The listing builds one solid part. Answer for the finished solid, in the listing's coordinates (mm). Face numbers are marked on the shaded views. A direction names the side the tool comes from. Round coordinates to 2 decimals unless told otherwise and drop trailing zeros. Write each loop counter-clockwise with the first axis right and the second up, starting at its lowest first coordinate (ties: lowest second). Pieces come first, ordered by that corner, then holes. Notation, with made-up numbers: (-15, 62.25) - (26, 62.25) arc R14 cw to (26, 82.25) - close; hole circle Ø5 at (43, 19.5). An arc over 180 degrees is marked (long way). Use a Markdown table: item, result. Add a question column.
1) A cutting plane is placed at D-D (y = 32.5). Give the vertices of the cut face in (x, z), then the cut area to 3 significant figures.
2) A cutting plane is placed at A-A (z = 9.75). Give the vertices of the cut face in (x, y), then the cut area to 3 significant figures.
3) Each of these flat-tipped pins is pushed along its axis until it touches: P1, Ø2.5, axis at y = 46.38, z = 14.3, coming from the -X side; P2, Ø1.8, axis at y = -14.12, z = 4.8, coming from the +X side; P3, Ø1.9, axis at y = -5.5, z = 25, coming from the -X side; P4, Ø0.8, axis at x = -25.5, z = 2, coming from the -Y side. Where does it stop, or does it pass through?
4) Determine the mould class of the marked faces 1, 2, 3 and 4 for opening direction Z: +Z half, -Z half, draft (parallel to the pull), parting line (faces both ways), or undercut.
5) A tool of negligible diameter and unlimited length cuts with its end or side. For the marked faces 5, 6, 7, 8 and 9, from which of +Z, -Z, +X, -X, +Y, -Y can it reach the whole face along a straight path? Write none if from no direction.
6) A cutting plane is placed at C-C (x = -21.5). Give the vertices of the cut face in (y, z).
7) A cutting plane is placed at B-B (x = -1). Give the vertices of the cut face in (y, z).
8) Find the intervals of material crossed by probe 1 along Y at (x, z) = (8, 24.6); probe 2 along Y at (x, z) = (-19.75, 23.8); probe 3 along X at (y, z) = (16.5, 25), in increasing order. Write a range as from..to.
```python
from build123d import *

# Parameters (mm, degrees)
EXTRUDE_1_DEPTH     = 28.6
SKETCH_1_R          = 6.5
CUT_EXTRUDE_1_DEPTH = 70.103002637
SKETCH_2_R          = 0.8
CUT_EXTRUDE_2_DEPTH = 70.103002637
CUT_EXTRUDE_4_DEPTH = 6
EXTRUDE_2_DEPTH     = 1.6
FILLET_1_R          = 1.5
FILLET_2_R          = 1.5
SKETCH_6_R          = 1.5
SKETCH_6_R_2        = 1.25
CUT_EXTRUDE_7_DEPTH = 8
CUT_EXTRUDE_8_DEPTH = 8


with BuildPart() as part:
    # Model → 凸台-拉伸1 (new body)
    with BuildSketch(Plane.XY):
        Polygon((-24.978787879, -17.92321671), (-14.678787879, -17.92321671), (-14.678787879, 24.376794113), (11.321212121, 24.376794113), (11.321212121, 51.376794114), (8.321212121, 51.376794114), (8.321212121, 28.376794114), (-23.578787879, 28.376794114), (-26.578787879, 25.376794114), (-26.578787879, 24.376794113), (-24.978787879, 24.376794113), align=None)
    extrude(amount=EXTRUDE_1_DEPTH)

    # 草图1 → 切除-拉伸1 (cut, through all)
    with BuildSketch(Plane.ZY.offset(24.978787879)):
        with Locations((14.3, -3.623205886)):
            Circle(SKETCH_1_R)
    extrude(amount=-CUT_EXTRUDE_1_DEPTH, mode=Mode.SUBTRACT)

    # 草图2 → 切除-拉伸2 (cut, through all)
    with BuildSketch(Plane.ZY.offset(24.978787879)):
        with Locations((23.8, 6.876794114)):
            Circle(SKETCH_2_R)
        with Locations((23.8, -14.123205886)):
            Circle(SKETCH_2_R)
        with Locations((4.8, -14.123205886)):
            Circle(SKETCH_2_R)
        with Locations((4.8, 6.876794114)):
            Circle(SKETCH_2_R)
    extrude(amount=-CUT_EXTRUDE_2_DEPTH, mode=Mode.SUBTRACT)

    # 草图3 → 切除-拉伸4 (cut)
    with BuildSketch(Plane.ZY.offset(24.978787879)):
        Polygon((6.3, -35.623205886), (22.3, -35.623205886), (22.3, -9.623205886), (24.3, -9.623205886), (24.3, 2.376794114), (22.3, 2.376794114), (22.3, 14.376794114), (6.3, 14.376794114), (6.3, 2.376794114), (4.3, 2.376794114), (4.3, -9.623205886), (6.3, -9.623205886), align=None)
    extrude(amount=-CUT_EXTRUDE_4_DEPTH, mode=Mode.SUBTRACT)

    # 草图5 → 凸台-拉伸2 (add, through all)
    with BuildSketch(Plane.ZY.offset(24.978787879)):
        Polygon((0, 24.376794113), (28.6, 24.376794113), (28.6, 10.676804938), (22.3, 10.676804938), (22.3, 14.376794114), (6.3, 14.376794114), (6.3, 10.676804938), (0, 10.676804938), align=None)
    extrude(amount=EXTRUDE_2_DEPTH)

    # 圆角1
    fillet_1_edges = [part.edges().sort_by_distance(p)[0] for p in [
        (-21.978787879, -9.623205886, 4.3),
        (-21.978787879, 2.376794114, 4.3),
        (-21.978787879, 2.376794114, 24.3),
        (-21.978787879, -9.623205886, 24.3),
    ]]
    fillet(fillet_1_edges, radius=FILLET_1_R)

    # 圆角2
    fillet_2_edges = [part.edges().sort_by_distance(p)[0] for p in [
        (-22.778787879, 14.376794114, 6.3),
        (-22.778787879, 14.376794114, 22.3),
    ]]
    fillet(fillet_2_edges, radius=FILLET_2_R)

    # 草图6 → 切除-拉伸7 (cut)
    with BuildSketch(Plane(origin=(11.321212121, 0, 0), x_dir=(0, 0, -1), z_dir=(1, 0, 0))):
        with Locations((-14.3, 46.376794114)):
            Circle(SKETCH_6_R)
        with Locations((-14.3, 26.376794113)):
            Circle(SKETCH_6_R_2)
        with Locations((-24.6, 26.376794113)):
            Circle(SKETCH_6_R_2)
        with Locations(Location((-4, 26.376794113, 0), (0, 0, 180))):
            Circle(SKETCH_6_R_2)
    extrude(amount=-CUT_EXTRUDE_7_DEPTH, mode=Mode.SUBTRACT)

    # 草图8 → 切除-拉伸8 (cut)
    with BuildSketch(Plane.ZY.offset(-8.321212121)):
        Polygon((8.3, 51.376794114), (0, 28.376794114), (-7.058670234, 55.306274643), align=None)
        Polygon((28.6, 28.376794114), (35.658670234, 55.306274643), (20.3, 51.376794114), align=None)
    extrude(amount=-CUT_EXTRUDE_8_DEPTH, mode=Mode.SUBTRACT)

    # M3 螺纹孔1: read off the stored shape, not the designer's step
    # M3 螺纹孔1 outline → M3 螺纹孔1 (revolve, cut)
    with BuildSketch(Plane(origin=(0, 26.376794113, 4), x_dir=(0, 1, 0), z_dir=(0, 0, -1))):
        Polygon((0, -7.429863653), (1.25, -6.678787879), (1.25, 3.046212121), (1.525, 3.321212121), (0, 3.321212121), align=None)
    revolve(axis=Axis((0, 26.376794113, 4), (1, 0, 0)), mode=Mode.SUBTRACT)

    # Hole Wizard M3 _1 2 outline → Hole Wizard M3 _1 2 (revolve, cut)
    with BuildSketch(Plane(origin=(0, 26.376794113, 14.3), x_dir=(0, 1, 0), z_dir=(0, 0, -1))):
        Polygon((1.25, 11.321212121), (1.25, 11.046212121), (1.525, 11.321212121), align=None)
        Polygon((1.25, 1.321212121), (1.25, 11.046212121), (0, 11.046212121), (0, 0.570136347), align=None)
    revolve(axis=Axis((0, 26.376794113, 14.3), (1, 0, 0)), mode=Mode.SUBTRACT)

    # Hole Wizard M3 _1 3 outline → Hole Wizard M3 _1 3 (revolve, cut)
    with BuildSketch(Plane(origin=(0, 26.376794113, 24.6), x_dir=(0, 1, 0), z_dir=(0, 0, -1))):
        Polygon((1.25, 11.321212121), (1.25, 11.046212121), (1.525, 11.321212121), align=None)
        Polygon((1.25, 1.321212121), (1.25, 3.321212121), (0, 3.321212121), (0, 0.570136347), align=None)
    revolve(axis=Axis((0, 26.376794113, 24.6), (1, 0, 0)), mode=Mode.SUBTRACT)


solid = part.part
```
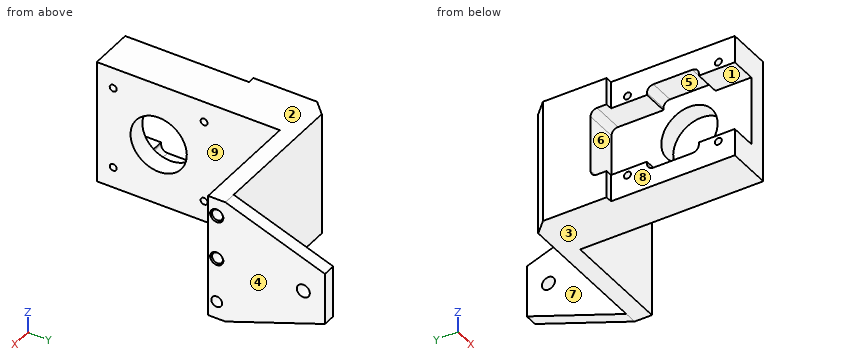
Entries:
| question | item | result |
|---|---|---|
| 1 | outline | (8.32, 1.49) - (11.32, 1.49) - (11.32, 27.11) - (8.32, 27.11) - close |
| 1 | area | 76.9 mm² |
| 2 | outline | (-26.58, 14.38) - (-18.98, 14.38) - (-18.98, 1.02) - (-14.68, 1.02) - (-14.68, 24.38) - (11.32, 24.38) - (11.32, 51.38) - (8.32, 51.38) - (8.32, 28.38) - (-23.58, 28.38) - (-26.58, 25.38) - close; (-18.98, -17.92) - (-14.68, -17.92) - (-14.68, -8.27) - (-18.98, -8.27) - close |
| 2 | area | 434 mm² |
| 3 | P1 | passes through |
| 3 | P2 | stops at x = -14.68 |
| 3 | P3 | stops at x = -24.98 |
| 3 | P4 | stops at y = 10.68 |
| 4 | face 1 | undercut |
| 4 | face 2 | +Z half |
| 4 | face 3 | -Z half |
| 4 | face 4 | draft |
| 5 | face 5 | -X |
| 5 | face 6 | -X, -Y |
| 5 | face 7 | +Z, -Z, -X, +Y |
| 5 | face 8 | +Z, -Z, -X, -Y |
| 5 | face 9 | +Z, -Z, +X, -Y |
| 6 | outline | (-17.92, 0) - (28.38, 0) - (28.38, 28.6) - (-17.92, 28.6) - (-17.92, 22.3) - (-9.62, 22.3) - (-9.62, 22.8) arc R1.5 cw to (-8.12, 24.3) - (0.88, 24.3) arc R1.5 cw to (2.38, 22.8) - (2.38, 22.3) - (12.88, 22.3) arc R1.5 cw to (14.38, 20.8) - (14.38, 7.8) arc R1.5 cw to (12.88, 6.3) - (2.38, 6.3) - (2.38, 5.8) arc R1.5 cw to (0.88, 4.3) - (-8.12, 4.3) arc R1.5 cw to (-9.62, 5.8) - (-9.62, 6.3) - (-17.92, 6.3) - close; hole circle Ø1.6 at (-14.12, 4.8); hole circle Ø1.6 at (-14.12, 23.8); hole circle Ø1.6 at (6.88, 4.8); hole circle Ø1.6 at (6.88, 23.8) |
| 7 | outline | (24.38, 0) - (28.38, 0) - (28.38, 28.6) - (24.38, 28.6) - close; hole circle Ø2.5 at (26.38, 4) |
| 8 | probe 1 | y = 24.38..25.13, 27.63..28.38 |
| 8 | probe 2 | y = -17.92..-14.92, -13.32..-9.24, 1.99..6.08, 7.68..28.38 |
| 8 | probe 3 | x = -26.58..-14.68 |
